CAD build for the part. Positions are in the model's coordinates, mm. A direction names the side the tool comes from. Coordinates: 2 decimals unless noted, no trailing zeros. Write each loop counter-clockwise with the first axis right and the second up, starting at its lowest first coordinate (ties: lowest second). Pieces come first, ordered by that corner, then holes. Notation, with made-up numbers: (11.25, 55.5) - (29.25, 55.5) arc R14 ccw to (29.25, 59.5) - close; hole circle Ø8 at (-17.5, 29). An arc over 180 degrees is marked (long way). Answer in a Markdown table with one row per item. Add a question column.
Q1. Band-saw the part on A-A (x = -18.5). List the corners of the cut face in (y, z), and give its area (3 significant figures).
Q2. Band-saw the part on C-C (z = 5). List the corners of the cut face in (x, y).
Q3. Two-plate mould, pull along X, no slides. Class faces 3 (the flat face through (31, -1, 1)), 4 (the flat face through (-30, -2, 1)), 5 (the flat face through (7, -1, 0)), 6 (the flat face through (0, -1, 1)): +X half, -X half, draft (parallel to the pull), parting line (faces both ways), or undercut.
Q4. Drill centre lines: line 1 along Y through (x, z) = (10, 1.25); line 2 along Y through (x, z) = (7, 12.5); line 3 along Z through (x, y) = (-14.5, -2.5). Where is each one in solid material? Low to high. Write a range as from..to.
Q5. Pin check, flat tips, straight feed: pin 1 (6 mm diameter, centred on x = -7.5, y = -3, fed in from +Z); pin 2 (0.8 mm diameter, centred on y = -35.5, z = 11.5, fed in from -X); pin 3 (5 mm diameter, centred on x = 0.5, y = -30.5, fed in from +Z). Stop position of each tip, or through.
Q6. 3-axis set-ups, long thin cutter, end or side, ignore diameter. For faces 1 (the flat face through (-1, -17, -1)), 2 (the flat face through (0, -27, 0)): which of +Z, -Z, +X, -X, +Y, -Y reach the whole face in a straight line?
Q7. Band-saw the part on B-B (y = -13.5). List the corners of the cut face in (x, z), and give its area (3 significant figures).
Q8. Band-saw the part on D-D (x = 0). List the corners of the cut face in (y, z), and give its area (3 significant figures).
Autodesk Fusion 360 part; units mm, degrees
sketch "Sketch1" plane through (0, 0, 0) normal (0, 0, 1) x (1, 0, 0)
  line L0 (-30, 15) -> (31, 15)
  line L1 (31, 15) -> (31, -18)
  line L2 (31, -18) -> (-30, -18)
  line L3 (-30, -18) -> (-30, 15)
  line L4 (-29.48, 14.4823) -> (30.5108, 14.4823)
  line L5 (30.5108, 14.4823) -> (30.5108, -17.4715)
  line L6 (30.5108, -17.4715) -> (-29.48, -17.4715)
  line L7 (-29.48, -17.4715) -> (-29.48, 14.4823)
extrude "Extrude1" add sketch "Sketch1" along normal blind 1.3
sketch "Sketch2" plane through (0, 0, 0) normal (0, 0, 1) x (1, 0, 0)
  line L0 (30.5108, -17.4715) -> (-29.48, -17.4715)
  line L1 (-29.48, -17.4715) -> (-29.48, 14.4823)
  line L2 (-29.48, 14.4823) -> (30.5108, 14.4823)
  line L3 (30.5108, 14.4823) -> (30.5108, -17.4715)
  point P0 (30.5108, -17.4715)
  point P1 (-29.48, 14.4823)
extrude "Extrude2" add sketch "Sketch2" along normal blind 1
sketch "Sketch3" plane through (0, 0, 0) normal (0, 0, -1) x (1, 0, 0)
  line L0 (31, 18) -> (-30, 18)
  line L1 (-30, 18) -> (-30, -15)
  line L2 (-30, -15) -> (31, -15)
  line L3 (31, -15) -> (31, 18)
  line L4 (5, -5) -> (-5, -5)
  line L5 (-5, -5) -> (-5, 35)
  line L6 (-5, 35) -> (5, 35)
  line L7 (5, 35) -> (5, -5)
extrude "Extrude3" add sketch "Sketch3" along normal blind 1 contours L0 L4 L5 L7 | L0 L5 L6 L7
sketch "Sketch4" plane through (0, 0, 0) normal (0, 0, -1) x (1, 0, 0)
  line L0 (-5, -5) -> (-5, 18)
  line L1 (-5, 18) -> (-30, 18)
  line L2 (-30, 18) -> (-30, -15)
  line L3 (-30, -15) -> (31, -15)
  line L4 (31, -15) -> (31, 18)
  line L5 (31, 18) -> (5, 18)
  line L6 (5, 18) -> (5, -5)
  line L7 (5, -5) -> (-5, -5)
sketch "Sketch5" plane through (0, 0, 0) normal (0, 1, 0) x (1, 0, 0)
sketch "Sketch6" plane through (0, 0, 1) normal (0, 0, 1) x (-1, 0, 0)
  line L0 (-30.5108, -14.4823) -> (29.48, -14.4823)
  line L1 (29.48, -14.4823) -> (29.48, 17.4715)
  line L2 (29.48, 17.4715) -> (-30.5108, 17.4715)
  line L3 (-30.5108, 17.4715) -> (-30.5108, -14.4823)
  line L4 (20, 11) -> (-20, 11) construction
  line L5 (-20, 11) -> (-20, -10) construction
  line L6 (-20, -10) -> (20, -10) construction
  line L7 (20, -10) -> (20, 11) construction
  dimension "d7" = 5
sketch "Sketch7" plane through (0, 0, 0) normal (1, 0, 0) x (0, 1, 0)
sketch "Sketch8" plane through (0, 0, 0) normal (0, 0, 1) x (1, 0, 0)
  line L0 (-14, -35) -> (13, -35)
  line L1 (13, -35) -> (13, -36)
  line L2 (13, -36) -> (-14, -36)
  line L3 (-14, -36) -> (-14, -35)
extrude "Extrude4" add sketch "Sketch8" along normal blind 17
extrude "Extrude5" add 1 faces at (-2, -35.6667, 0) along direction (0, 0, -1) blind 1
extrude "Extrude6" add 1 faces at (13, -35.3333, 11) along direction (1, 0, 0) blind 1
Checked values:
| question | item | result |
|---|---|---|
| 1 | outline | (-18, 0) - (15, 0) - (15, 1.3) - (14.48, 1.3) - (14.48, 1) - (-17.47, 1) - (-17.47, 1.3) - (-18, 1.3) - close |
| 1 | area | 33.3 mm² |
| 2 | outline | (-14, -36) - (14, -36) - (14, -35) - (-14, -35) - close |
| 3 | face 3 | +X half |
| 3 | face 4 | -X half |
| 3 | face 5 | draft |
| 3 | face 6 | undercut |
| 4 | line 1 | y = -36..-35, -18..-17.47, 14.48..15 |
| 4 | line 2 | y = -36..-35 |
| 4 | line 3 | z = 0..1 |
| 5 | pin 1 | stops at z = 1 |
| 5 | pin 2 | stops at x = -14 |
| 5 | pin 3 | stops at z = 0 |
| 6 | face 1 | -Z, +X, -X, +Y, -Y |
| 6 | face 2 | +Z, +X, -X |
| 7 | outline | (-30, 0) - (-5, 0) - (-5, -1) - (5, -1) - (5, 0) - (31, 0) - (31, 1.3) - (30.51, 1.3) - (30.51, 1) - (-29.48, 1) - (-29.48, 1.3) - (-30, 1.3) - close |
| 7 | area | 71.3 mm² |
| 8 | outline | (-36, -1) - (5, -1) - (5, 0) - (15, 0) - (15, 1.3) - (14.48, 1.3) - (14.48, 1) - (-17.47, 1) - (-17.47, 1.3) - (-18, 1.3) - (-18, 0) - (-35, 0) - (-35, 17) - (-36, 17) - close |
| 8 | area | 91.3 mm² |
